For this review, take the finished solid that the model builds, in its own axes (mm). Face numbers are marked on the shaded views. Round coordinates to 2 decimals unless told otherwise and drop trailing zeros. Write each loop counter-clockwise with the first axis right and the second up, starting at its lowest first coordinate (ties: lowest second). Pieces come first, ordered by that corner, then holes. Notation, with made-up numbers: (49.25, -1.75) -> (100.25, -1.75) arc R9 ccw to (100.25, 14.25) -> close; hole circle Ø7 at (63, 45). An arc over 180 degrees is marked (long way). Answer as CSV lines item,"result". Start each with the question number.
Item 1: Mouldability with a two-part tool opening along X and no side actions: class the marked faces 1, 2 and 3 as +X half, -X half, draft (parallel to the pull), parting line (faces both ways), or undercut.
Item 2: Take a section at C-C on x = 3.5. Give the boundary of the cut face in (y, z).
Item 3: For pin 1 Ø5 at (x, z) = (-2, 13) entering from -Y; pin 2 Ø2 at (x, y) = (-1, 2.5) entering from +Z; pin 3 Ø6 at (x, z) = (-0.5, 18.5) entering from -Y, all flat-tipped, find the tip position at first contact; note any pin that passes through.
Item 4: Wall thickness on probe 1 along X at (y, z) = (0.6, 11); probe 2 along X at (y, z) = (2, 28.5); probe 3 along Z at (x, y) = (-5.75, 1.05): over which ranges is each line inside the solid? List them lowest first. Write a range as from..to.
Item 5: Take a section at D-D on x = -4. Give the boundary of the cut face in (y, z).
Item 6: Take a section at B-B on y = 0.65. Give the boundary of the cut face in (x, z), then the cut area to 3 significant figures.
Item 7: Take a section at A-A on z = 9. Give the boundary of the cut face in (x, y).
```python
from build123d import *

# Parameters (mm, degrees)
F1_DEPTH = 30
F3_DEPTH = 1


with BuildPart() as f1:
    # F0 (on Top) → F1 (new body)
    with BuildSketch(Plane.XY):
        with BuildLine():
            Line((-10, 3), (-10, 0))
            Line((-10, 0), (-8, 0))
            Line((-8, 0), (-8, 1))
            Line((-8, 1), (-9, 1))
            Line((-9, 1), (-9, 2.323808))
            ThreePointArc((-9, 2.323808), (0, 4), (9, 2.323808))
            Line((9, 2.323808), (9, 1))
            Line((9, 1), (8, 1))
            Line((8, 1), (8, 0))
            Line((8, 0), (10, 0))
            Line((10, 0), (10, 3))
            ThreePointArc((10, 3), (0, 5), (-10, 3))
        make_face()
    extrude(amount=F1_DEPTH)

    # F2 (on face) → F3 (join)
    with BuildSketch(Plane(origin=(0, 0, 0), x_dir=(1, 0, 0), z_dir=(0, 0, -1))):
        with BuildLine():
            Line((10, 0), (-10, 0))
            Line((-10, 0), (-10, -3))
            ThreePointArc((-10, -3), (0, -5), (10, -3))
            Line((10, -3), (10, 0))
        make_face()
    extrude(amount=-F3_DEPTH)


solid = f1.part
```
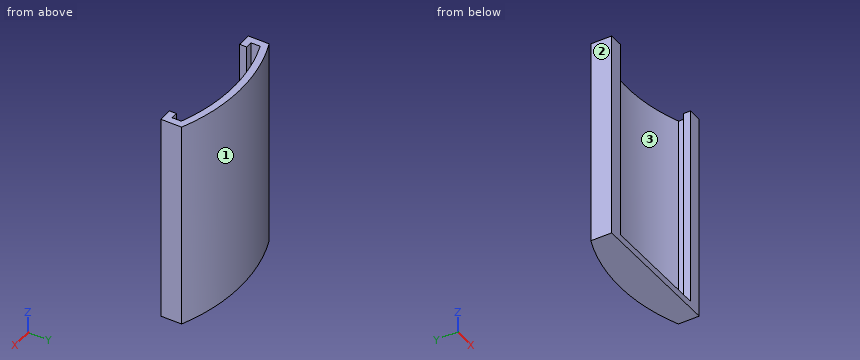
Output values:
1,face 1,"parting line"
1,face 2,"-X half"
1,face 3,"undercut"
2,outline,"(0, 0) -> (4.76, 0) -> (4.76, 30) -> (3.75, 30) -> (3.75, 1) -> (0, 1) -> close"
3,pin 1,"stops at y = 3.59"
3,pin 2,"stops at z = 1"
3,pin 3,"stops at y = 3.75"
4,probe 1,"x = -10..-8, 8..10"
4,probe 2,"x = -10..-9, 9..10"
4,probe 3,"z = 0..1"
5,outline,"(0, 0) -> (4.69, 0) -> (4.69, 30) -> (3.68, 30) -> (3.68, 1) -> (0, 1) -> close"
6,outline,"(-10, 0) -> (10, 0) -> (10, 30) -> (8, 30) -> (8, 1) -> (-8, 1) -> (-8, 30) -> (-10, 30) -> close"
6,area,"136 mm^2"
7,outline,"(-10, 0) -> (-8, 0) -> (-8, 1) -> (-9, 1) -> (-9, 2.32) arc R25 cw to (9, 2.32) -> (9, 1) -> (8, 1) -> (8, 0) -> (10, 0) -> (10, 3) arc R26 ccw to (-10, 3) -> close"
